```python
from build123d import *

# Parameters (mm, degrees)
SKETCH1_R                = 6.3
SKETCH1_R_2              = 4.2
BOSS_EXTRUDE1_DEPTH      = 16
BOSS_EXTRUDE1_DEPTH_BACK = 16
SKETCH2_R                = 1.3
CUT_EXTRUDE1_DEPTH       = 14
CUT_EXTRUDE1_DEPTH_BACK  = 10
SKETCH3_R                = 4.2
SKETCH3_R_2              = 3.7
BOSS_EXTRUDE2_DEPTH      = 4


with BuildPart() as part:
    # Sketch1 → Boss-Extrude1 (new body, two sides)
    with BuildSketch(Plane.XY) as boss_extrude1_sk:
        Circle(SKETCH1_R)
        Circle(SKETCH1_R_2, mode=Mode.SUBTRACT)
    extrude(amount=BOSS_EXTRUDE1_DEPTH)
    extrude(boss_extrude1_sk.sketch, amount=-BOSS_EXTRUDE1_DEPTH_BACK)

    # Sketch2 → Cut-Extrude1 (cut, two sides)
    with BuildSketch(Plane(origin=(0, 0, 0), x_dir=(0, 0, -1), z_dir=(1, 0, 0))) as cut_extrude1_sk:
        with Locations((-4, 0)):
            Circle(SKETCH2_R)
        with Locations((8, 0)):
            Circle(SKETCH2_R)
    extrude(amount=CUT_EXTRUDE1_DEPTH, mode=Mode.SUBTRACT)
    extrude(cut_extrude1_sk.sketch, amount=-CUT_EXTRUDE1_DEPTH_BACK, mode=Mode.SUBTRACT)

    # Sketch3 → Boss-Extrude2 (add)
    with BuildSketch(Plane.XY.offset(16)):
        Circle(SKETCH3_R)
        Circle(SKETCH3_R_2, mode=Mode.SUBTRACT)
    extrude(amount=-BOSS_EXTRUDE2_DEPTH)


solid = part.part
```
Geometry: final body of the model. Coordinates: model frame, mm. A direction names the side the tool comes from. Coordinates: 2 decimals unless noted, no trailing zeros. Order: outer loops, then holes, each group sorted by start corner. A loop starts at its lowest first (then second) coordinate and runs counter-clockwise, first axis right, second up. Notation, with made-up numbers: M 8.5,77.5 L 64.5,77.5 A28 cw 64.5,111.5 Z; hole C 24,-32 d3. An arc over 180 degrees is marked long. Answer in a Markdown table with one row per item. Add a question column.
Q1. Mould query, pull axis X, two halves, no side actions, for faces 1 (the cylindrical face through (5.13, 0.39, -9.24)), 2 (the cylindrical face through (3.88, -1.61, -1.8)), 3 (the cylindrical face through (5.82, -2.41, 0.22)). Classes: released by +X, released by -X, zero draft, split by the parting line, or undercut.
Q2. Section query B-B on x = 0. Return the cut outline in (y, z), and give its area (3 significant figures).
Q3. Section query D-D on z = 4. Return the cut outline in (x, y).
Q4. Section query A-A on y = 0. Return the cut outline in (x, z).
Q5. Contact query for a flat-ended pin moving along its axis: P1, Ø2, axis at x = -1.5, z = 5.5, coming from the +Y side. Output: stop coordinate, or through.
Q6. Line query: L1, parallel to Z at x = 5.15, y = 0; L2, parallel to Y at x = 4.7, z = 4; L3, parallel to Y at x = 0, z = 13.8. Output: solid intervals per line, ascending.
Q7. Section query C-C on z = -3. Return the cut outline in (x, y), and give its area (3 significant figures).
Q8. Reachability of faces 4 (the cylindrical face through (-0.802, -3.612, 14.028)), 5 (the flat face through (0, -4, 12)) from +Z, -Z, +X, -X, +Y, -Y: full face, straight path, thin tool, end or side. Return the list, or none.
Completed:
| question | item | result |
|---|---|---|
| 1 | face 1 | zero draft |
| 1 | face 2 | undercut |
| 1 | face 3 | split by the parting line |
| 2 | outline | M -6.3,-16 L -4.2,-16 L -4.2,12 L -3.7,12 L -3.7,16 L -6.3,16 Z; M 3.7,12 L 4.2,12 L 4.2,-16 L 6.3,-16 L 6.3,16 L 3.7,16 Z |
| 2 | area | 138 mm2 |
| 3 | outline | M -6.16,-1.3 A6.3 ccw 6.16,-1.3 L 3.99,-1.3 A4.2 cw -3.99,-1.3 Z; M -6.16,1.3 L -3.99,1.3 A4.2 cw 3.99,1.3 L 6.16,1.3 A6.3 ccw Z |
| 4 | outline | M -6.3,-16 L -4.2,-16 L -4.2,-9.3 L -6.3,-9.3 Z; M -6.3,-6.7 L -4.2,-6.7 L -4.2,2.7 L -6.3,2.7 Z; M -6.3,5.3 L -4.2,5.3 L -4.2,12 L -3.7,12 L -3.7,16 L -6.3,16 Z; M 3.7,12 L 4.2,12 L 4.2,5.3 L 6.3,5.3 L 6.3,16 L 3.7,16 Z; M 4.2,-16 L 6.3,-16 L 6.3,-9.3 L 4.2,-9.3 Z; M 4.2,-6.7 L 6.3,-6.7 L 6.3,2.7 L 4.2,2.7 Z |
| 5 | P1 | stops at y = 6.28 |
| 6 | L1 | z = -16 to -9.3, -6.7 to 2.7, 5.3 to 16 |
| 6 | L2 | y = -4.2 to -1.3, 1.3 to 4.2 |
| 6 | L3 | y = -6.3 to -3.7, 3.7 to 6.3 |
| 7 | outline | C 0,0 d12.6; hole C 0,0 d8.4 |
| 7 | area | 69.3 mm2 |
| 8 | face 4 | +Z, -Z |
| 8 | face 5 | -Z |
